```python
from build123d import *

# Parameters (mm, degrees)
F1_DEPTH = 1
F2_W     = 16
F2_H     = 21
F2_W_2   = 14
F2_H_2   = 19
F3_DEPTH = 3
F4_W     = 14
F4_H     = 19
F5_DEPTH = 1


with BuildPart() as f1:
    # F0 (on Top) → F1 (new body)
    with BuildSketch(Plane.XY):
        with BuildLine():
            ThreePointArc((12.5, 13), (11.914214, 14.414214), (10.5, 15))
            Line((10.5, 15), (-10.5, 15))
            ThreePointArc((-10.5, 15), (-11.914214, 14.414214), (-12.5, 13))
            Line((-12.5, 13), (-12.5, -13))
            ThreePointArc((-12.5, -13), (-11.914214, -14.414214), (-10.5, -15))
            Line((-10.5, -15), (10.5, -15))
            ThreePointArc((10.5, -15), (11.914214, -14.414214), (12.5, -13))
            Line((12.5, -13), (12.5, 13))
        make_face()
    extrude(amount=F1_DEPTH)

    # F2 (on face) → F3 (join)
    with BuildSketch(Plane.XY.offset(1)):
        Rectangle(F2_W, F2_H)
        Rectangle(F2_W_2, F2_H_2, mode=Mode.SUBTRACT)
    extrude(amount=F3_DEPTH)

    # F4 (on face) → F5 (join)
    with BuildSketch(Plane.XY.offset(4)):
        with BuildLine():
            ThreePointArc((12.5, 13), (11.914214, 14.414214), (10.5, 15))
            Line((10.5, 15), (-10.5, 15))
            ThreePointArc((-10.5, 15), (-11.914214, 14.414214), (-12.5, 13))
            Line((-12.5, 13), (-12.5, -13))
            ThreePointArc((-12.5, -13), (-11.914214, -14.414214), (-10.5, -15))
            Line((-10.5, -15), (10.5, -15))
            ThreePointArc((10.5, -15), (11.914214, -14.414214), (12.5, -13))
            Line((12.5, -13), (12.5, 13))
        make_face()
        Rectangle(F4_W, F4_H, mode=Mode.SUBTRACT)
    extrude(amount=F5_DEPTH)


solid = f1.part
```
The model under review builds one solid part; all positions refer to its coordinate system, in mm. A direction names the side the tool comes from. Give positions to 0.01 mm unless a question says otherwise; leave off trailing zeros. Order: outer loops, then holes, each group sorted by start corner. A loop starts at its lowest first (then second) coordinate and runs counter-clockwise, first axis right, second up. Notation, with made-up numbers: (-19.5, 51.5) - (-13.5, 51.5) arc R18 ccw to (-13.5, 58.5) - close; hole circle Ø5 at (29, 24). An arc over 180 degrees is marked (long way). Use CSV: the item, a comma, the result in double quotes. Start each with the question number.
Q1. Tool access review of faces 1 (the flat face through (-7, 0, 3)), 2 (the flat face through (-8, 0, 2)), 3 (the flat face through (0, 0, 0)), 4 (the flat face through (8, 0, 2)), 5 (the flat face through (0, 10.5, 2)): name each direction out of +Z, -Z, +X, -X, +Y, -Y from which nothing blocks a thin tool from reaching the whole face with its end or side.
Q2. The part is to be moulded in two halves that separate along Y. For faces 6 (the flat face through (7, 0, 3)), 7 (the cylindrical face through (11.9, -14.43, 4.49)), 8 (the flat face through (12.5, -0.2, 0.5)), say which applies: +Y half, -Y half, draft (parallel to the pull), parting line (faces both ways), or undercut.
Q3. We need section D-D, the plane x = -2. Write out the cut boundary in (y, z).
Q4. We need section C-C, the plane y = 9. Write out the cut boundary in (x, z).
Q5. We need section B-B, the plane z = 2.85. Write out the cut boundary in (x, y), and give its area (3 significant figures).
Q6. Clearance check with flat-ended pins moving along their axes: pin 1 Ø0.9 at (y, z) = (1.5, 3) entering from +X; pin 2 Ø1.5 at (y, z) = (-4, 2) entering from -X; pin 3 Ø0.9 at (x, z) = (-0.5, 2.5) entering from +Y. State where each tip first meets the part, or that it passes through.
Q7. We need section A-A, the plane x = -8.75. Write out the cut boundary in (y, z).
Q8. To check wall thickness, follow line 1 along Y through (x, z) = (-2.5, 3.1); line 2 along X through (y, z) = (-3.5, 2.65); line 3 along Z through (x, y) = (10.5, 7). State the ranges of each line that lie inside material, in increasing order. Write a range as [from, to].
Outcome:
1,face 1,"+Z"
1,face 2,"-X, +Y, -Y"
1,face 3,"-Z, +X, -X, +Y, -Y"
1,face 4,"+X, +Y, -Y"
1,face 5,"+X, -X, +Y"
2,face 6,"undercut"
2,face 7,"-Y half"
2,face 8,"draft"
3,outline,"(-15, 0) - (15, 0) - (15, 1) - (10.5, 1) - (10.5, 4) - (15, 4) - (15, 5) - (9.5, 5) - (9.5, 1) - (-9.5, 1) - (-9.5, 5) - (-15, 5) - (-15, 4) - (-10.5, 4) - (-10.5, 1) - (-15, 1) - close"
4,outline,"(-12.5, 0) - (12.5, 0) - (12.5, 1) - (8, 1) - (8, 4) - (12.5, 4) - (12.5, 5) - (7, 5) - (7, 1) - (-7, 1) - (-7, 5) - (-12.5, 5) - (-12.5, 4) - (-8, 4) - (-8, 1) - (-12.5, 1) - close"
5,outline,"(-8, -10.5) - (8, -10.5) - (8, 10.5) - (-8, 10.5) - close; hole (-7, -9.5) - (7, -9.5) - (7, 9.5) - (-7, 9.5) - close"
5,area,"70.0 mm^2"
6,pin 1,"stops at x = 8"
6,pin 2,"stops at x = -8"
6,pin 3,"stops at y = 10.5"
7,outline,"(-15, 0) - (15, 0) - (15, 1) - (-15, 1) - close; (-15, 4) - (15, 4) - (15, 5) - (-15, 5) - close"
8,line 1,"y = [-10.5, -9.5], [9.5, 10.5]"
8,line 2,"x = [-8, -7], [7, 8]"
8,line 3,"z = [0, 1], [4, 5]"
